```python
from build123d import *

# Parameters (mm, degrees)
SKETCH2_W                 = 15
SKETCH2_H                 = 30
BOSS_EXTRUDE1_DEPTH       = 2.5
SKETCH3_R                 = 2.5
BOSS_EXTRUDE2_DEPTH       = 10
FILLET3_R                 = 2.5
FILLET4_R                 = 2.5
F_3_0MM_DOWEL_HOLE1_D     = 3
F_3_0MM_DOWEL_HOLE1_DEPTH = 12
F_3_0MM_DOWEL_HOLE1_TIP   = 0.901290929


with BuildPart() as part:
    # Sketch2 → Boss-Extrude1 (new body)
    with BuildSketch(Plane(origin=(0, 0, 0), x_dir=(1, 0, 0), z_dir=(0, 1, 0))):
        with Locations((-7.5, 15)):
            Rectangle(SKETCH2_W, SKETCH2_H)
    extrude(amount=BOSS_EXTRUDE1_DEPTH)

    # Sketch3 → Boss-Extrude2 (add)
    with BuildSketch(Plane.XY):
        with BuildLine():
            ThreePointArc((-13.75, 1.25), (-11.25, -1.25), (-8.75, 1.25))
            Line((-8.75, 1.25), (-13.75, 1.25))
        make_face()
        with BuildLine():
            Line((-13.75, 1.25), (-8.75, 1.25))
            ThreePointArc((-8.75, 1.25), (-11.25, 3.75), (-13.75, 1.25))
        make_face()
        with Locations(Location((-3.75, 1.25, 0), (0, 0, 150))):
            Circle(SKETCH3_R)
    extrude(amount=BOSS_EXTRUDE2_DEPTH)

    # Fillet3
    fillet3_edges = [part.edges().sort_by_distance(p)[0] for p in [
        (-13.75, 1.25, 10),
    ]]
    fillet(fillet3_edges, radius=FILLET3_R)

    # Fillet4
    fillet4_edges = [part.edges().sort_by_distance(p)[0] for p in [
        (-1.584936491, 0, 10),
    ]]
    fillet(fillet4_edges, radius=FILLET4_R)

    # Ø3.0mm Dowel Hole1
    with Locations(Plane(origin=(0, 2.5, 0), x_dir=(1, 0, 0), z_dir=(0, 1, 0))):
        with Locations((-7.5, 18.71)):
            Hole(F_3_0MM_DOWEL_HOLE1_D / 2, depth=F_3_0MM_DOWEL_HOLE1_DEPTH)
            with Locations((0, 0, -(F_3_0MM_DOWEL_HOLE1_DEPTH + F_3_0MM_DOWEL_HOLE1_TIP / 2))):  # 118° drill point
                Cone(0, F_3_0MM_DOWEL_HOLE1_D / 2, F_3_0MM_DOWEL_HOLE1_TIP, mode=Mode.SUBTRACT)


solid = part.part
```
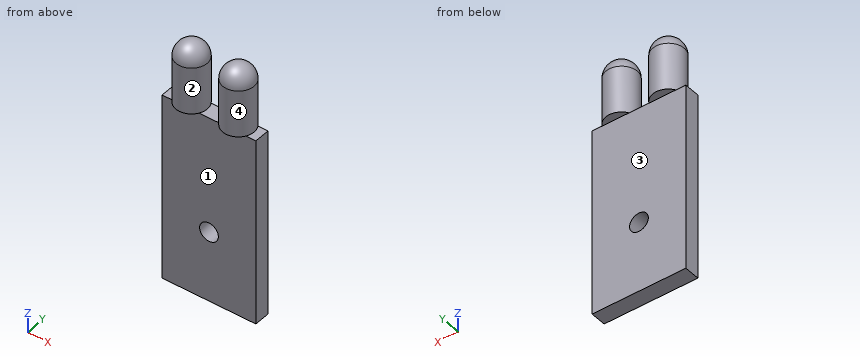
Source: CAD feature listing. Evaluate the final solid. Frame: model axes, mm. Face numbers are marked on the shaded views. A direction names the side the tool comes from. Coordinates: 2 decimals unless noted, no trailing zeros. Loops run counter-clockwise (first coordinate to the right, second up) from the corner with the lowest first, then second, coordinate; pieces in that order, holes last. Notation, with made-up numbers: M -16,9 L 7,9 A15 ccw 7,17 Z; hole C 86,-36.5 d2. An arc over 180 degrees is marked long. Put each result on its own line as item: value. Start each with the question number.
1) Contact query for flat-ended pins moving along their axis: pin 1 Ø4 at (x, z) = (-6, -15.5) entering from +Y; pin 2 Ø1.7 at (x, y) = (-1, 1.5) entering from +Z; pin 3 Ø0.6 at (x, y) = (-4.5, 3) entering from -Z. Output: stop coordinate, or through.
2) Cut plane A-A on x = -7.5. Return the cut outline in (y, z).
3) Cut plane D-D on x = -3.75. Return the cut outline in (y, z), then the cut area to 3 significant figures.
4) Reachability of the marked faces 3 and 4 from +Z, -Z, +X, -X, +Y, -Y: full face, straight path, thin tool, end or side. Return the list, or none.
5) Cut plane C-C on z = -18.71. Return the cut outline in (x, y), then the cut area to 3 significant figures.
6) Ray query, L1, parallel to X at y = 0.6, z = -18.71; L2, parallel to Z at x = -7.5, y = 1.2; L3, parallel to Y at x = -2.25, z = -15.5. Return the intervals inside material, ascending. Write a range as from..to.
7) Cut plane B-B on y = 1.25. Return the cut outline in (x, z), then the cut area to 3 significant figures.
8) Pull-direction query (X, two-part tool) for the marked faces 1 and 2; classes: pulls with the +X half, pulls with the -X half, needs draft (parallel to the pull), parting line crosses it, or undercut.
The answers:
1. pin 1: stops at y = 2.5
1. pin 2: stops at z = 9.11
1. pin 3: stops at z = 0
2. outline: M 0,-30 L 2.5,-30 L 2.5,-20.21 L 0,-20.21 Z; M 0,-17.21 L 2.5,-17.21 L 2.5,0 L 0,0 Z
3. outline: M -1.25,0 L 0,0 L 0,-30 L 2.5,-30 L 2.5,0 L 3.75,0 L 3.75,7.5 A2.5 ccw -1.25,7.5 Z
3. area: 122 mm²
4. face 3: -Z, +X, -X, +Y
4. face 4: +Z
5. outline: M -15,0 L -9,0 L -9,2.5 L -15,2.5 Z; M -6,0 L 0,0 L 0,2.5 L -6,2.5 Z
5. area: 30.0 mm²
6. L1: x = -15..-9, -6..0
6. L2: z = -30..-20.21, -17.21..0
6. L3: y = 0..2.5
7. outline: M -15,-30 L 0,-30 L 0,0 L -1.25,0 L -1.25,7.5 A2.5 ccw -6.25,7.5 L -6.25,0 L -8.75,0 L -8.75,7.5 A2.5 ccw -13.75,7.5 L -13.75,0 L -15,0 Z; hole C -7.5,-18.71 d3
7. area: 538 mm²
8. face 1: needs draft
8. face 2: undercut
